Autodesk Inventor part; units mm, degrees
ref_plane "YZ Plane" through (0, 0, 0) normal (1, 0, 0) x (0, 1, 0)
ref_plane "XZ Plane" through (0, 0, 0) normal (0, 1, 0) x (-1, 0, 0)
ref_plane "XY Plane" through (0, 0, 0) normal (0, 0, 1) x (1, 0, 0)
sketch "Boceto1" plane through (0, 0, -197.5) normal (1, 0, 0) x (0, 1, 0)
  arc A0 (10, 400) -> (-10, 400) centre (0, 400) ccw
  line L0 (-10, 400) -> (-15, 0)
  line L1 (10, 400) -> (15, 0)
  arc A1 (-14.9953, 0.3749) -> (14.9953, 0.3749) centre (0, 0) ccw
  circle A2 centre (0, 0) radius 5
  dimension "d1" = 20
  dimension "d0" = 10
extrude "Extrusión1" add sketch "Boceto1" along normal blind 3
properties part number "BrazoPalanca"
Geometry: final body of the model. Coordinates: model frame, mm. Coordinates: 2 decimals unless noted, no trailing zeros. Order: outer loops, then holes, each group sorted by start corner. A loop starts at its lowest first (then second) coordinate and runs counter-clockwise, first axis right, second up.
(1) First-contact query: pin 1 (8 mm diameter, centred on y = 0, z = -197.5, fed in from +X). Flat tip, straight axial feed; report the tip coordinate or a pass-through.
(2) Section query D-D (z = 75). Return the cut outline in (x, y).
(3) Material intervals for probe 1 along Z at (x, y) = (2.25, 0); probe 2 along Z at (x, y) = (2.4, -2.25); probe 3 along Z at (x, y) = (0.8, 9), sorted ascending.
(4) Section query C-C (z = -34.5). Return the cut outline in (x, y), plus the area to 3 significant figures.
(5) Section query B-B (x = 0.6). Return the cut outline in (y, z), plus the area to 3 significant figures.
(6) Section query A-A (y = 0). Return the cut outline in (x, z).
(7) Draft query along Y for faces 1 (the face through (1.5, -0.2, 212.5)), 2 (the face through (3, 0, 3)), 3 (the face through (1.479, -0.651, -202.457)). Return one class per face: pulls with the +Y half, pulls with the -Y half, needs draft (parallel to the pull), parting line crosses it, or undercut.
Solution:
1. pin 1: passes through
2. outline: (0, -11.59) - (3, -11.59) - (3, 11.59) - (0, 11.59) - close
3. probe 1: z = -212.5 to -202.5, -192.5 to 212.5
3. probe 2: z = -212.33 to -201.97, -193.03 to 212.24
3. probe 3: z = -209.5 to 206.86
4. outline: (0, -12.96) - (3, -12.96) - (3, 12.96) - (0, 12.96) - close
4. area: 77.8 mm2
5. outline: (-15, -197.5) arc R15 ccw to (15, -197.5) - (10, 202.5) arc R10 ccw to (-10, 202.5) - close; hole circle Ø10 at (0, -197.5)
5. area: 10,400 mm2
6. outline: (0, -212.5) - (3, -212.5) - (3, -202.5) - (0, -202.5) - close; (0, -192.5) - (3, -192.5) - (3, 212.5) - (0, 212.5) - close
7. face 1: parting line crosses it
7. face 2: needs draft
7. face 3: undercut
